Geometry: final body of the model. Coordinates: model frame, mm. A direction names the side the tool comes from. Round coordinates to 2 decimals unless told otherwise and drop trailing zeros. Return JSON: item names as keys, results as strings. Group by question number.
1. Material intervals for probe 1 along Z at (x, y) = (0, -1); probe 2 along X at (y, z) = (4.75, -18); probe 3 along Z at (x, y) = (0, -2.25), sorted ascending.
2. First-contact query: pin 1 Ø1 at (x, y) = (27.5, 3) entering from +Z; pin 2 Ø5 at (y, z) = (-2, -64.5) entering from -X; pin 3 Ø4 at (x, y) = (2, -3) entering from -Z. Flat tips, straight axial feed; report the tip coordinate or a pass-through.
3. Set-up query: faces 1 (the face through (-9.632, -0.07, -40.597)), 2 (the face through (9, 0, -50)), 3 (the face through (-6, 0, -72)), 4 (the face through (3.314, 5.986, -19.824)). Return all of +Z, -Z, +X, -X, +Y, -Y with unobstructed straight access to the full face (end or side cutting, diameter ignored); none if empty.
4. Draft query along X for faces 5 (the face through (19.941, -0.07, 26.564)), 6 (the face through (-9, 0, -50)), 7 (the face through (-12.87, -0.07, -7.39)). Return one class per face: +X half, -X half, draft (parallel to the pull), parting line (faces both ways), or undercut.
from build123d import *

# Parameters (mm, degrees)
PAD_DEPTH       = 7
CHAMFER_SIZE    = 2
CHAMFER001_SIZE = 2
SKETCH001_R     = 6.5
PAD001_DEPTH    = 14
FILLET_R        = 2
SKETCH002_R     = 6
PAD002_DEPTH    = 15
FILLET001_R     = 0.48


with BuildPart() as pad002:
    # Sketch → Pad (new body, symmetric)
    with BuildSketch(Plane.XZ):
        with BuildLine():
            ThreePointArc((10.524526, -6.744209), (3.513789, 11.99597), (-12.5, 0))
            Line((-12.5, 0), (-13.250923, -14.981192))
            ThreePointArc((-23.249077, -14.981192), (-18.25, -19.8851), (-13.250923, -14.981192))
            Line((-24, 0), (-23.249077, -14.981192))
            ThreePointArc((24.415762, -23.682477), (19.181941, 26.948774), (-24, 0))
            Line((24.072611, -23.949315), (24.415762, -23.682477))
            ThreePointArc((24.072611, -23.949315), (14.686334, -35.499894), (11.33, -50))
            Line((-11, -50), (11.33, -50))
            ThreePointArc((-5.784749, -32.195289), (-9.66936, -40.723598), (-11, -50))
            Line((-5.784749, -32.195289), (10.524526, -6.744209))
        make_face()
    extrude(amount=PAD_DEPTH, both=True)

    # Chamfer
    chamfer_edges = [pad002.edges().sort_by_distance(p)[0] for p in [
        (3.513789, -7, 11.99597),
    ]]
    chamfer(chamfer_edges, length=CHAMFER_SIZE)

    # Chamfer001
    chamfer001_edges = [pad002.edges().sort_by_distance(p)[0] for p in [
        (19.181941, 7, 26.948774),
    ]]
    chamfer(chamfer001_edges, length=CHAMFER001_SIZE)

    # Sketch001 → Pad001 (new body)
    with BuildSketch(Plane(origin=(0, 0, -50), x_dir=(1, 0, 0), z_dir=(0, 0, -1))):
        Circle(SKETCH001_R)
    extrude(amount=PAD001_DEPTH)

    # Fillet
    fillet_edges = [pad002.edges().sort_by_distance(p)[0] for p in [
        (-6.5, 0, -50),
    ]]
    fillet(fillet_edges, radius=FILLET_R)

    # Sketch002 → Pad002 (new body)
    with BuildSketch(Plane(origin=(0, 0, -64), x_dir=(1, 0, 0), z_dir=(0, 0, -1))):
        Circle(SKETCH002_R)
    extrude(amount=PAD002_DEPTH)


with BuildPart() as fillet001:
    # Sketch003 → Revolution (revolve)
    with BuildSketch(Plane.XZ):
        with BuildLine():
            Line((0, -63.291796), (0, -81.291796))
            ThreePointArc((0, -81.291796), (3.211399, -80.699347), (6, -79))
            Line((6, -65.583592), (6, -79))
            ThreePointArc((6, -65.583592), (3.211399, -63.884245), (0, -63.291796))
        make_face()
    revolve(axis=Axis((0, 0, 0), (0, 0, 1)))

    # Fusion: union Pad002
    add(pad002.part)

    # Fillet001
    fillet001_edges = [fillet001.edges().sort_by_distance(p)[0] for p in [
        (-6, 0, -64),
    ]]
    fillet(fillet001_edges, radius=FILLET001_R)


solid = fillet001.part
Taken from the geometry:
{
 "1": {"probe 1": "-81.24 to -23.17, 12.5 to 29.39", "probe 2": "-22.16 to -14.34, 3.31 to 30", "probe 3": "-81.01 to -23.17, 12.5 to 29.39"},
 "2": {"pin 1": "z = 21.42", "pin 2": "x = -6.5", "pin 3": "z = -81.15"},
 "3": {"face 1": "-X, +Y, -Y", "face 2": "-Z, +X", "face 3": "-Z", "face 4": "+Y"},
 "4": {"face 5": "parting line", "face 6": "draft", "face 7": "undercut"}
}
